Build history of the part. All positions in model axes, mm. Face numbers are marked on the shaded views. A direction names the side the tool comes from. Round coordinates to 2 decimals unless told otherwise and drop trailing zeros. Write each loop counter-clockwise with the first axis right and the second up, starting at its lowest first coordinate (ties: lowest second). Pieces come first, ordered by that corner, then holes.
Item 1: Wall check: probe 1 along X at (y, z) = (0.5, 0); probe 2 along Y at (x, z) = (9, 9.5); probe 3 along X at (y, z) = (6, 12). Give the ranges that are in metal, low to high.
Item 2: Mould opens along X. For the marked faces 3, 4 and 5 say: +X half, -X half, draft (parallel to the pull), parting line (faces both ways), or undercut.
Item 3: Band-saw the part on D-D, the plane z = 14. Write the cut outline in (x, y), then the cut area to 3 significant figures.
Item 4: Band-saw the part on B-B, the plane y = 10.25. Write the cut outline in (x, z).
Item 5: Band-saw the part on A-A, the plane x = -3.5. Write the cut outline in (y, z), then the cut area to 3 significant figures.
Item 6: Band-saw the part on C-C, the plane z = -15. Write the cut outline in (x, y), then the cut area to 3 significant figures.
Item 7: Drop flat-ended pins along their axis: pin 1 Ø3 at (x, z) = (0, 19.25) entering from -Y; pin 2 Ø1.5 at (x, y) = (-9, 8.5) entering from +Z; pin 3 Ø3 at (y, z) = (3, 4.5) entering from +X; pin 4 Ø2 at (y, z) = (8.5, 13) entering from -X. Give the stop position or say it passes through.
Item 8: 3-axis set-ups, long thin cutter, end or side, ignore diameter. For the marked faces 1 and 2: which of +Z, -Z, +X, -X, +Y, -Y reach the whole face in a straight line?
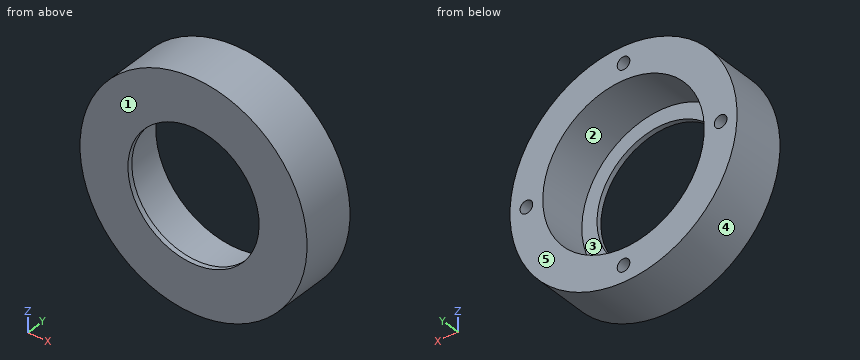
```python
from build123d import *

# Parameters (mm, degrees)
SKETCH_1_R          = 22.5
EXTRUDE_1_DEPTH     = 11
SKETCH_2_R          = 16
CUT_EXTRUDE_1_DEPTH = 10
SKETCH_3_R          = 13
CUT_EXTRUDE_2_DEPTH = 34.35416016
M3X0_51_D           = 2.5
M3X0_51_DEPTH       = 8.5
M3X0_51_TIP         = 0.751075774


with BuildPart() as part:
    # Эскиз1 → Бобышка-Вытянуть1 (new body)
    with BuildSketch(Plane(origin=(0, 0, 0), x_dir=(1, 0, 0), z_dir=(0, 1, 0))):
        with Locations(Location((0, 0, 0), (0, 0, 270))):
            Circle(SKETCH_1_R)
    extrude(amount=EXTRUDE_1_DEPTH)

    # Эскиз2 → Вырез-Вытянуть1 (cut)
    with BuildSketch(Plane(origin=(0, 11, 0), x_dir=(1, 0, 0), z_dir=(0, 1, 0))):
        with Locations(Location((0, 0, 0), (0, 0, 270))):
            Circle(SKETCH_2_R)
    extrude(amount=-CUT_EXTRUDE_1_DEPTH, mode=Mode.SUBTRACT)

    # Эскиз3 → Вырез-Вытянуть2 (cut, through all)
    with BuildSketch(Plane(origin=(0, 1, 0), x_dir=(1, 0, 0), z_dir=(0, 1, 0))):
        with Locations(Location((0, 0, 0), (0, 0, 270))):
            Circle(SKETCH_3_R)
    extrude(amount=-CUT_EXTRUDE_2_DEPTH, mode=Mode.SUBTRACT)

    # Отверстие обработанное метчиком M3x0.51
    with Locations(Plane(origin=(0, 11, 0), x_dir=(1, 0, 0), z_dir=(0, 1, 0))):
        with Locations((-19.25, 0), (0, -19.25), (19.25, 0), (0, 19.25)):
            Hole(M3X0_51_D / 2, depth=M3X0_51_DEPTH)
            with Locations((0, 0, -(M3X0_51_DEPTH + M3X0_51_TIP / 2))):  # 118° drill point
                Cone(0, M3X0_51_D / 2, M3X0_51_TIP, mode=Mode.SUBTRACT)


solid = part.part
```
Results:
1. probe 1: x = -22.5 to -13, 13 to 22.5
1. probe 2: y = 0 to 1
1. probe 3: x = -19.03 to -10.58, 10.58 to 19.03
2. face 3: undercut
2. face 4: parting line
2. face 5: draft
3. outline: (-17.61, 0) - (17.61, 0) - (17.61, 11) - (7.75, 11) - (7.75, 1) - (-7.75, 1) - (-7.75, 11) - (-17.61, 11) - close
3. area: 233 mm2
4. outline: circle Ø45 at (0, 0); hole circle Ø2.5 at (-19.25, 0); hole circle Ø32 at (0, 0); hole circle Ø2.5 at (0, -19.25); hole circle Ø2.5 at (0, 19.25); hole circle Ø2.5 at (19.25, 0)
5. outline: (0, -22.23) - (11, -22.23) - (11, -15.61) - (1, -15.61) - (1, -12.52) - (0, -12.52) - close; (0, 12.52) - (1, 12.52) - (1, 15.61) - (11, 15.61) - (11, 22.23) - (0, 22.23) - close
5. area: 152 mm2
6. outline: (-16.77, 0) - (16.77, 0) - (16.77, 11) - (5.57, 11) - (5.57, 1) - (-5.57, 1) - (-5.57, 11) - (-16.77, 11) - close
6. area: 258 mm2
7. pin 1: stops at y = 0
7. pin 2: stops at z = 20.93
7. pin 3: stops at x = 22.3
7. pin 4: stops at x = -19.03
8. face 1: +Z, -Z, +X, -X, -Y
8. face 2: +Y
